The drawing under review shows one solid part. Ordinate dimensions are in mm from its lowest x, y, z. Give positions to 0.01 mm unless a question says otherwise; leave off trailing zeros. Loops run counter-clockwise (first coordinate to the right, second up) from the corner with the lowest first, then second, coordinate; pieces in that order, holes last.
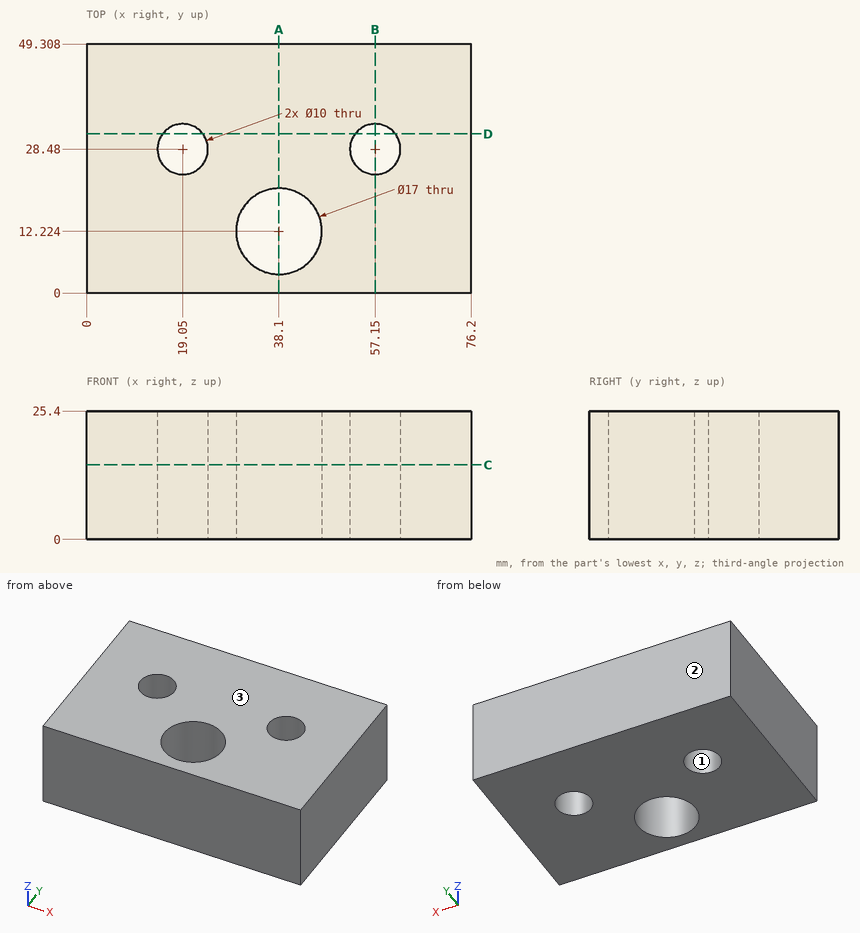
Item 1: Take a section at B-B on x = 57.15. Give the boundary of the cut face in (y, z), and give its area (3 significant figures).
Answer:
outline: (0, 0) - (23.48, 0) - (23.48, 25.4) - (0, 25.4) - close; (33.48, 0) - (49.31, 0) - (49.31, 25.4) - (33.48, 25.4) - close
area: 998 mm2
Item 2: The part is to be moulded in two halves that separate along Y. For the marked faces 1, 2 and 3, say which applies: released by +Y, released by -Y, zero draft, split by the parting line, or undercut.
Answer:
face 1: undercut
face 2: released by +Y
face 3: zero draft
Item 3: Clearance check with a flat-ended pin moving along its axis: pin 1 Ø6 at (x, y) = (19.05, 28.48) entering from -Z. State where the tip first meets the part, or that it passes through.
Answer:
pin 1: passes through
Item 4: For L1, parallel to X at y = 26, z = 4.5; L2, parallel to X at y = 27.5, z = 20.5; L3, parallel to Y at x = 19.05, z = 16, list the stretches that pass through material, from the lowest coordinate up.
Answer:
L1: x = 0 to 14.71, 23.39 to 52.81, 61.49 to 76.2
L2: x = 0 to 14.15, 23.95 to 52.25, 62.05 to 76.2
L3: y = 0 to 23.48, 33.48 to 49.31
Item 5: Take a section at A-A on x = 38.1. Give the boundary of the cut face in (y, z), and give its area (3 significant figures).
Answer:
outline: (0, 0) - (3.72, 0) - (3.72, 25.4) - (0, 25.4) - close; (20.72, 0) - (49.31, 0) - (49.31, 25.4) - (20.72, 25.4) - close
area: 821 mm2
Item 6: Take a section at C-C on z = 14.75. Give the boundary of the cut face in (x, y), and give its area (3 significant figures).
Answer:
outline: (0, 0) - (76.2, 0) - (76.2, 49.31) - (0, 49.31) - close; hole circle Ø10 at (19.05, 28.48); hole circle Ø17 at (38.1, 12.22); hole circle Ø10 at (57.15, 28.48)
area: 3,370 mm2
Item 7: Take a section at D-D on y = 31.5. Give the boundary of the cut face in (x, z), and give its area (3 significant figures).
Answer:
outline: (0, 0) - (15.07, 0) - (15.07, 25.4) - (0, 25.4) - close; (23.03, 0) - (53.17, 0) - (53.17, 25.4) - (23.03, 25.4) - close; (61.13, 0) - (76.2, 0) - (76.2, 25.4) - (61.13, 25.4) - close
area: 1,530 mm2
